Verification items for the finished model (mm, model axes). A direction names the side the tool comes from. Coordinates: 2 decimals unless noted, no trailing zeros. Order: outer loops, then holes, each group sorted by start corner. A loop starts at its lowest first (then second) coordinate and runs counter-clockwise, first axis right, second up. Notation, with made-up numbers: (-17, 72.25) -> (42, 72.25) arc R33 cw to (42, 110.25) -> close; hole circle Ø6 at (-28.5, 77). An arc over 180 degrees is marked (long way). Write each question's results on one line, items separated by ' | '. Start each with the question number.
(1) Draft check along X on faces 1 (the flat face through (-2, 24.424, 3)), 2 (the cylindrical face through (29.31, 69.4, 2.54)), 3 (the cylindrical face through (8.761, 41.594, 2.535)), 4 (the cylindrical face through (-19.55, 0.6, 2.54)). Enter one of: +X half, -X half, draft (parallel to the pull), parting line (faces both ways), or undercut.
(2) Cross-section at B-B on x = 20.5. Enter the section's corners in (y, z).
(3) Cross-section at D-D on z = 9. Enter the section's corners in (x, y).
(4) Go/stop test with flat-tipped pins: pin 1 (4 mm diameter, centred on x = 7, z = 2.5, fed in from -Y); pin 2 (1.5 mm diameter, centred on x = -8, y = 11.5, fed in from +Z); pin 3 (5 mm diameter, centred on x = 17.5, z = 16, fed in from -Y). Record where each tip stops, or that it passes through.
(5) Cross-section at A-A on y = 38.5. Enter the section's corners in (x, z).
(6) Cross-section at C-C on y = 6. Enter the section's corners in (x, z).
(7) Set-up check for faces 5 (the flat face through (-2, 45.424, 3)), 6 (the cylindrical face through (25.22, 3.89, 12.89)), 7 (the flat face through (5, 0, 2)): record each of +Z, -Z, +X, -X, +Y, -Y from which the full face is reachable in a straight line by a thin tool's end or side.
(8) Thickness scan on probe 1 along X at (y, z) = (33, 1); probe 2 along Z at (x, y) = (0, 41); probe 3 along Y at (x, z) = (-13, 5.75). Record the ranges inside material, lowest first. Write a range as [from, to].
Autodesk Inventor part; units mm, degrees
ref_plane "YZ Plane" through (0, 0, 0) normal (1, 0, 0) x (0, 1, 0)
ref_plane "XZ Plane" through (0, 0, 0) normal (0, 1, 0) x (-1, 0, 0)
ref_plane "XY Plane" through (0, 0, 0) normal (0, 0, 1) x (1, 0, 0)
sketch "Skizze1" plane through (0, 0, 0) normal (0, 0, 1) x (1, 0, 0)
  line L0 (-20.1198, 0) -> (29.8802, 0)
  line L1 (29.8802, 0) -> (29.8802, 70)
  line L2 (29.8802, 70) -> (-20.1198, 70)
  line L3 (-20.1198, 70) -> (-20.1198, 0)
  point P0 (0, 0)
  dimension "d0" = 50
  dimension "d1" = 70
extrude "Extrusion1" add sketch "Skizze1" along normal blind 5
fillet "Rundung1" radius 2 4 edges at (-20.1198, 0, 2.5) (29.8802, 0, 2.5) (29.8802, 70, 2.5) (-20.1198, 70, 2.5)
sketch "Skizze2" plane through (0, 0, 5) normal (0, 0, 1) x (1, 0, 0)
  line L0 (-3.9308, 24.4243) -> (-0.9308, 24.4243)
  line L1 (-0.9308, 24.4243) -> (-0.9308, 45.4243)
  line L2 (-0.9308, 45.4243) -> (-3.9308, 45.4243)
  line L3 (-3.9308, 45.4243) -> (-3.9308, 24.4243)
  point P0 (0, 0)
  dimension "d5" = 3
  dimension "d6" = 21
extrude "Extrusion2" cut sketch "Skizze2" against normal up to surface (5 mm away)
sketch "Skizze3" plane through (0, 0, 5) normal (0, 0, 1) x (1, 0, 0)
  line L0 (-20.1198, 2) -> (-20.1198, 68)
  line L1 (27.8802, 0) -> (-18.1198, 0)
  line L2 (29.8802, 68) -> (29.8802, 2)
  line L3 (-18.1198, 70) -> (27.8802, 70)
  line L4 (-3.9308, 45.4243) -> (10.5692, 45.4243)
  line L5 (10.5692, 45.4243) -> (10.5692, 24.4243)
  line L6 (10.5692, 24.4243) -> (-3.9308, 24.4243)
  line L7 (-3.9308, 24.4243) -> (-3.9308, 45.4243)
  circle A0 centre (8.0692, 42.9243) radius 1.5
  circle A1 centre (8.0692, 26.9243) radius 1.5
  circle A2 centre (21.7604, 34.9243) radius 2.5
  circle A3 centre (-14.1198, 64) radius 2.5
  circle A4 centre (23.8802, 64) radius 2.5
  circle A5 centre (-14.1198, 6) radius 2.5
  circle A6 centre (23.8802, 6) radius 2.5
  point P0 (0, 0)
  dimension "d9" = 14.5
  dimension "d10" = 21
  dimension "d11" = 3
  dimension "d12" = 3
  dimension "d13" = 2.5
  dimension "d14" = 2.5
  dimension "d15" = 2.5
  dimension "d16" = 2.5
  dimension "d17" = 5
  dimension "d18" = 5
  dimension "d19" = 5
  dimension "d20" = 5
  dimension "d21" = 5
  dimension "d22" = 6
  dimension "d23" = 6
  dimension "d24" = 6
  dimension "d25" = 6
  dimension "d26" = 6
  dimension "d27" = 6
  dimension "d28" = 6
  dimension "d29" = 6
sketch "Skizze4" plane through (0, 0, 5) normal (0, 0, 1) x (1, 0, 0)
  circle A0 centre (-14.1198, 64) radius 2.5
  circle A1 centre (23.8802, 64) radius 2.5
  circle A2 centre (-14.1198, 6) radius 2.5
  circle A3 centre (23.8802, 6) radius 2.5
  point P0 (0, 0)
  dimension "d30" = 5
  dimension "d31" = 5
  dimension "d32" = 5
  dimension "d33" = 5
extrude "Extrusion3" add sketch "Skizze4" along normal blind 16
extrude "Extrusion4" cut sketch "Skizze3" against normal up to surface (5 mm away) contours A0 | A1 | A2
properties part number "Platte"
Results are:
1) face 1: undercut | face 2: +X half | face 3: undercut | face 4: -X half
2) outline: (0, 0) -> (32.77, 0) -> (32.77, 5) -> (0, 5) -> close; (37.08, 0) -> (70, 0) -> (70, 5) -> (37.08, 5) -> close
3) outline: circle Ø5 at (-14.12, 6); circle Ø5 at (-14.12, 64); circle Ø5 at (23.88, 6); circle Ø5 at (23.88, 64)
4) pin 1: stops at y = 0 | pin 2: stops at z = 5 | pin 3: passes through
5) outline: (-20.12, 0) -> (-3.93, 0) -> (-3.93, 5) -> (-20.12, 5) -> close; (-0.93, 0) -> (29.88, 0) -> (29.88, 5) -> (-0.93, 5) -> close
6) outline: (-20.12, 0) -> (29.88, 0) -> (29.88, 5) -> (26.38, 5) -> (26.38, 21) -> (21.38, 21) -> (21.38, 5) -> (-11.62, 5) -> (-11.62, 21) -> (-16.62, 21) -> (-16.62, 5) -> (-20.12, 5) -> close
7) face 5: +Z, -Z | face 6: +Z | face 7: +Z, -Z, +X, -X, -Y
8) probe 1: x = [-20.12, -3.93], [-0.93, 20.16], [23.36, 29.88] | probe 2: z = [0, 5] | probe 3: y = [3.76, 8.24], [61.76, 66.24]
